Verification items for the finished model (mm, model axes). Coordinates: 2 decimals unless noted, no trailing zeros. Order: outer loops, then holes, each group sorted by start corner. A loop starts at its lowest first (then second) coordinate and runs counter-clockwise, first axis right, second up. Notation, with made-up numbers: M 74,4.5 L 82,4.5 A31 cw 82,39.5 Z; hole C 32.5,-11.75 d2. An arc over 180 degrees is marked long. Answer as a JSON object with one key per item and string values. Group by question number.
(1) Cross-section at C-C (z = 1.55). Enter the section's corners in (x, y).
(2) Cross-section at B-B (y = 7.5). Enter the section's corners in (x, z).
(3) Material ranges on line 1 (Y direction, x = -7, z = 1.25); line 2 (X direction, y = -7, z = 1.2); line 3 (Y direction, x = 0, z = 0.1), recorded low to high.
(4) Cross-section at A-A (x = -16.5). Enter the section's corners in (y, z), plus the area to 3 significant figures.
Autodesk Inventor part; units mm, degrees
ref_plane "YZ Plane" through (0, 0, 0) normal (1, 0, 0) x (0, 1, 0)
ref_plane "XZ Plane" through (0, 0, 0) normal (0, 1, 0) x (-1, 0, 0)
ref_plane "XY Plane" through (0, 0, 0) normal (0, 0, 1) x (1, 0, 0)
sketch "Sketch1" plane through (0, 0, 0) normal (0, 0, 1) x (1, 0, 0)
  line L0 (-35.35, 0) -> (35.35, 0) construction
  line L1 (0, -35.35) -> (0, 35.35) construction
  line L2 (-25.25, 25.25) -> (25.25, 25.25)
  line L3 (25.25, 25.25) -> (25.25, -25.25)
  line L4 (25.25, -25.25) -> (-25.25, -25.25)
  line L5 (-25.25, -25.25) -> (-25.25, 25.25)
  line L6 (-18, 12) -> (18, 12)
  line L7 (18, 12) -> (18, -12)
  line L8 (18, -12) -> (-18, -12)
  line L9 (-18, -12) -> (-18, 12)
  point P0 (0, 0)
  point P1 (0, 25.25)
  point P2 (25.25, 0)
  point P3 (0, 12)
  point P4 (18, 0)
  dimension "d0" = 50.5
  dimension "d1" = 50.5
  dimension "d2" = 36
  dimension "d3" = 24
extrude "Extrusion1" add sketch "Sketch1" along normal blind 2.5
fillet "Fillet1" radius 2 4 edges at (-25.25, -25.25, 1.25) (25.25, -25.25, 1.25) (-25.25, 25.25, 1.25) (25.25, 25.25, 1.25)
fillet "Fillet2" radius 0.5 16 edges at (24.6642, -24.6642, 2.5) (25.25, 0, 2.5) (24.6642, 24.6642, 2.5) (0, 25.25, 2.5) (-24.6642, 24.6642, 2.5) (-25.25, 0, 2.5) (-24.6642, -24.6642, 2.5) (0, -25.25, 2.5) (-24.6642, -24.6642, 0) (-25.25, 0, 0) (-24.6642, 24.6642, 0) (0, 25.25, 0) (24.6642, 24.6642, 0) (25.25, 0, 0) (24.6642, -24.6642, 0) (0, -25.25, 0)
equation "\"d1\" = d0"
properties part number "F114DiaReseau"
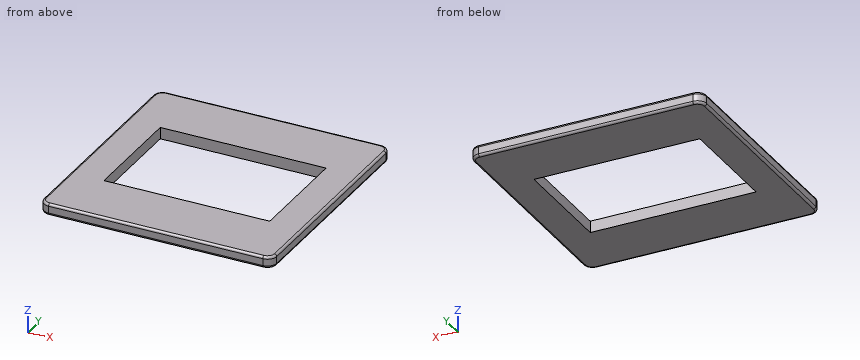
Taken from the geometry:
{
 "1": {"outline": "M -25.25,-23.25 A2 ccw -23.25,-25.25 L 23.25,-25.25 A2 ccw 25.25,-23.25 L 25.25,23.25 A2 ccw 23.25,25.25 L -23.25,25.25 A2 ccw -25.25,23.25 Z; hole M -18,-12 L 18,-12 L 18,12 L -18,12 Z"},
 "2": {"outline": "M -25.25,0.5 A0.5 ccw -24.75,0 L -18,0 L -18,2.5 L -24.75,2.5 A0.5 ccw -25.25,2 Z; M 18,0 L 24.75,0 A0.5 ccw 25.25,0.5 L 25.25,2 A0.5 ccw 24.75,2.5 L 18,2.5 Z"},
 "3": {"line 1": "y = -25.25 to -12, 12 to 25.25", "line 2": "x = -25.25 to -18, 18 to 25.25", "line 3": "y = -25.05 to -12, 12 to 25.05"},
 "4": {"outline": "M -25.25,0.5 A0.5 ccw -24.75,0 L -12,0 L -12,2.5 L -24.75,2.5 A0.5 ccw -25.25,2 Z; M 12,0 L 24.75,0 A0.5 ccw 25.25,0.5 L 25.25,2 A0.5 ccw 24.75,2.5 L 12,2.5 Z", "area": "66.0 mm²"}
}
